Answer from the drawing. Dimensions are ordinates in mm from the lowest x, y and z of the part. A direction names the side the tool comes from. Coordinates: 2 decimals unless noted, no trailing zeros. Write each loop counter-clockwise with the first axis right and the second up, starting at its lowest first coordinate (ties: lowest second). Pieces come first, ordered by that corner, then holes.
(1) The part is cut by section C-C, the plane y = 415.5. Determine the outline of the cut face in (x, z), and give its area (3 significant figures).
(2) The part is cut by section D-D, the plane z = 37. Determine the outline of the cut face in (x, y), and give its area (3 significant figures).
(3) Determine the mould class of the marked faces 1, 2 and 3 for opening direction Z: pulls with the +Z half, pulls with the -Z half, needs draft (parallel to the pull), parting line crosses it, or undercut.
(4) Which of the six approach directions +Z, -Z, +X, -X, +Y, -Y give full straight-line access (tool end or side, diameter ignored) to the marked faces 4, 5, 6 and 7?
(5) The part is cut by section B-B, the plane z = 234. Determine the outline of the cut face in (x, y).
(6) Straight lines are drawn through the part: line 1 along Z through (x, y) = (85, 154.5); line 2 along Z through (x, y) = (410.5, 438.5); line 3 along Y through (x, z) = (173, 83). For each, find the intervals that lie inside material, in ascending order.
(7) The part is cut by section A-A, the plane x = 408. Determine the outline of the cut face in (y, z).
(8) Given pin 1 (6 mm diameter, centred on x = 409, y = 299, fed in from +Z); pin 2 (6 mm diameter, centred on x = 344.5, y = 449, fed in from +Z); pin 3 (22.5 mm diameter, centred on x = 34.5, z = 23.5, fed in from +Y); pin 4 (12 mm diameter, centred on y = 110.5, z = 213, fed in from +X), each flat-ended and moving along its own axis, determine where each tip first touches the part or whether it passes through.
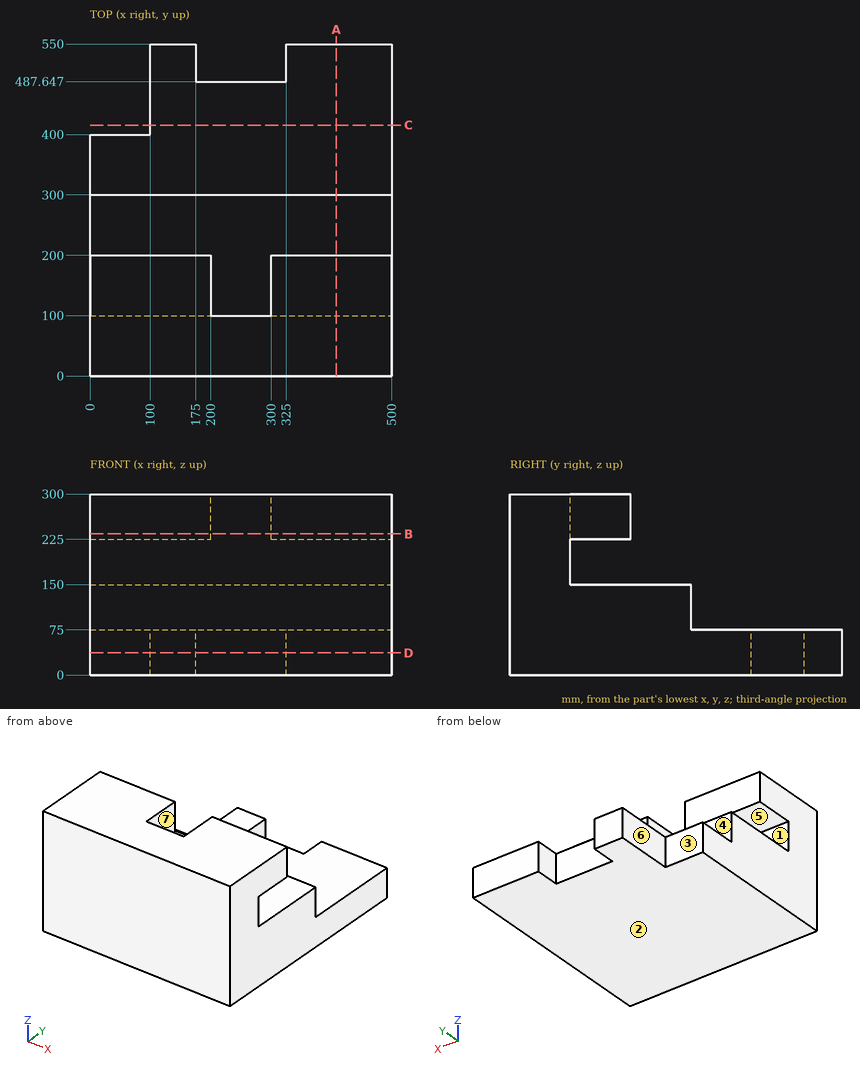
Computed:
1. outline: (100, 0) - (500, 0) - (500, 75) - (100, 75) - close
1. area: 30,000 mm2
2. outline: (0, 0) - (500, 0) - (500, 550) - (325, 550) - (325, 487.65) - (175, 487.65) - (175, 550) - (100, 550) - (100, 400) - (0, 400) - close
2. area: 251,000 mm2
3. face 1: undercut
3. face 2: pulls with the -Z half
3. face 3: needs draft
4. face 4: +Z, +X, -X, +Y
4. face 5: +X, -X, +Y
4. face 6: +Z, -Z, -X, +Y
4. face 7: +Z, +Y
5. outline: (0, 0) - (500, 0) - (500, 200) - (300, 200) - (300, 100) - (200, 100) - (200, 200) - (0, 200) - close
6. line 1: z = 0 to 150, 225 to 300
6. line 2: z = 0 to 75
6. line 3: y = 0 to 300
7. outline: (0, 0) - (550, 0) - (550, 75) - (300, 75) - (300, 150) - (100, 150) - (100, 225) - (200, 225) - (200, 300) - (0, 300) - close
8. pin 1: stops at z = 150
8. pin 2: stops at z = 75
8. pin 3: stops at y = 400
8. pin 4: passes through
